CAD build for the part. Positions are in the model's coordinates, mm. Round coordinates to 2 decimals unless told otherwise and drop trailing zeros. Loops run counter-clockwise (first coordinate to the right, second up) from the corner with the lowest first, then second, coordinate; pieces in that order, holes last.
Autodesk Inventor part; units mm, degrees
ref_plane "YZ Plane" through (0, 0, 0) normal (1, 0, 0) x (0, 1, 0)
ref_plane "XZ Plane" through (0, 0, 0) normal (0, 1, 0) x (-1, 0, 0)
ref_plane "XY Plane" through (0, 0, 0) normal (0, 0, 1) x (1, 0, 0)
sketch "Sketch1" plane through (0, 0, 0) normal (0, 1, 0) x (-1, 0, 0)
  line L0 (-15, -10) -> (15, -10)
  line L1 (15, -10) -> (15, 10)
  line L2 (15, 10) -> (-15, 10)
  line L3 (-15, 10) -> (-15, -10)
  line L4 (-15, -10) -> (15, 10) construction
  line L5 (15, -10) -> (-15, 10) construction
  circle A0 centre (5, 0) radius 2
  circle A1 centre (-5, 0) radius 2
  point P0 (0, 0)
  dimension "d0" = 30
  dimension "d1" = 20
  dimension "d2" = 4
  dimension "d3" = 4
extrude "Extrusion1" add sketch "Sketch1" along normal blind 1
properties part number "trail 10"
Item 1: Cut at B-B (z = 0). List the corners of the cut face in (x, y).
Verdict:
outline: (-15, 0) - (-7, 0) - (-7, 1) - (-15, 1) - close; (-3, 0) - (3, 0) - (3, 1) - (-3, 1) - close; (7, 0) - (15, 0) - (15, 1) - (7, 1) - close
Item 2: Mould opens along X. For faces 1 (the flat face through (0.2, 0.5, -10)), 2 (the flat face through (15, 0.5, 0.1)), 3 (the cylindrical face through (-3.002, 0.493, -0.088)) say: released by +X, released by -X, zero draft, split by the parting line, or undercut.
Verdict:
face 1: zero draft
face 2: released by +X
face 3: undercut
Item 3: Wall check: L1, parallel to Z at x = 5, y = 0.35; L2, parallel to Z at x = -3.5, y = 0.5. Give the ranges that are in metal, low to high.
Verdict:
L1: z = -10 to -2, 2 to 10
L2: z = -10 to -1.32, 1.32 to 10
Item 4: Cut at A-A (x = -5). List the corners of the cut face in (y, z), plus the area to 3 significant figures.
Verdict:
outline: (0, -10) - (1, -10) - (1, -2) - (0, -2) - close; (0, 2) - (1, 2) - (1, 10) - (0, 10) - close
area: 16.0 mm2
Item 5: Cut at C-C (y = 0.55). List the corners of the cut face in (x, z).
Verdict:
outline: (-15, -10) - (15, -10) - (15, 10) - (-15, 10) - close; hole circle Ø4 at (-5, 0); hole circle Ø4 at (5, 0)
